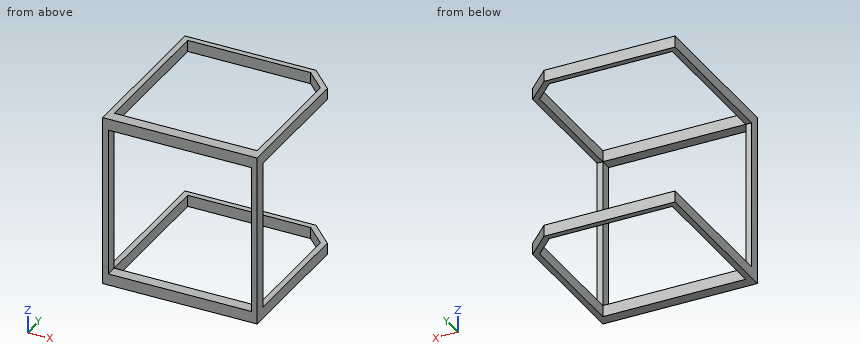
from build123d import *

# Parameters (mm, degrees)
BOSS_EXTRUDE1_DEPTH = 40
SKETCH2_W           = 20
SKETCH2_H           = 40
BOSS_EXTRUDE2_DEPTH = 520


with BuildPart() as part:
    # Sketch1 → Boss-Extrude1 (new body)
    with BuildSketch(Plane.XY):
        Polygon((0, 0), (0, 560), (458.284271247, 560), (540, 478.284271247), (540, 0), align=None)
        Polygon((20, 40), (20, 540), (450, 540), (520, 470), (520, 40), align=None, mode=Mode.SUBTRACT)
    boss_extrude1 = extrude(amount=BOSS_EXTRUDE1_DEPTH)

    # Sketch2 → Boss-Extrude2 (add)
    with BuildSketch(Plane.XY.offset(40)):
        with Locations((530, 20)):
            Rectangle(SKETCH2_W, SKETCH2_H)
        with Locations((10, 20)):
            Rectangle(SKETCH2_W, SKETCH2_H)
    extrude(amount=BOSS_EXTRUDE2_DEPTH)

    # Mirror1: Boss-Extrude1 across plane
    add(boss_extrude1.mirror(Plane(origin=(0, 0, 300), x_dir=(1, 0, 0), z_dir=(0, 0, -1))))


solid = part.part
Could you check a few things on this model? Use its own coordinates, in mm. Give positions to 0.01 mm unless a question says otherwise; leave off trailing zeros. Write each loop counter-clockwise with the first axis right and the second up, starting at its lowest first coordinate (ties: lowest second). Pieces come first, ordered by that corner, then holes. Notation, with made-up numbers: (-33.5, 31.25) -> (-14.5, 31.25) arc R13 cw to (-14.5, 56.25) -> close; hole circle Ø4 at (86, 42). An arc over 180 degrees is marked (long way). Write each question's results on one line, items separated by ' | '. Start each with the question number.
Q1. Suppose I cut it at A-A, the plane x = 352. List the corners of the cut face in (y, z) for me.
Q2. I need wall thicknesses on probe 1 along X at (y, z) = (37, 459.5); probe 2 along Y at (x, z) = (392.5, 567.5); probe 3 along X at (y, z) = (473, 30). Which ranges of each line are inside material? Lowest first, please.
Q3. I'm going to push flat-ended pins straight in: pin 1 Ø12 at (x, y) = (193.5, 29) entering from -Z; pin 2 Ø6 at (x, z) = (15, 352.5) entering from +Y. Where does each tip first touch, or does it pass through?
Q4. Suppose I cut it at B-B, the plane z = 540.5. List the corners of the cut face in (x, y) for me, and give its area (3 significant figures).
Q5. Suppose I cut it at C-C, the plane y = 190. List the corners of the cut face in (x, z) for me, and give its area (3 significant figures).
Outcome:
1) outline: (0, 0) -> (40, 0) -> (40, 40) -> (0, 40) -> close; (0, 560) -> (40, 560) -> (40, 600) -> (0, 600) -> close; (540, 0) -> (560, 0) -> (560, 40) -> (540, 40) -> close; (540, 560) -> (560, 560) -> (560, 600) -> (540, 600) -> close
2) probe 1: 0 to 20, 520 to 540 | probe 2: 0 to 40, 540 to 560 | probe 3: 0 to 20, 517 to 540
3) pin 1: z = 0 | pin 2: y = 40
4) outline: (0, 0) -> (20, 0) -> (20, 40) -> (0, 40) -> close; (520, 0) -> (540, 0) -> (540, 40) -> (520, 40) -> close | area: 1,600 mm2
5) outline: (0, 0) -> (20, 0) -> (20, 40) -> (0, 40) -> close; (0, 560) -> (20, 560) -> (20, 600) -> (0, 600) -> close; (520, 0) -> (540, 0) -> (540, 40) -> (520, 40) -> close; (520, 560) -> (540, 560) -> (540, 600) -> (520, 600) -> close | area: 3,200 mm2
